Input: dimensioned drawing with shaded views. Units: mm. Origin: part minimum x, y, z. A direction names the side the tool comes from. Round coordinates to 2 decimals unless told otherwise and drop trailing zeros. Loops run counter-clockwise (first coordinate to the right, second up) from the corner with the lowest first, then second, coordinate; pieces in that order, holes last. Notation, with made-up numbers: (-5.5, 58.5) - (21.5, 58.5) arc R19 ccw to (21.5, 95.5) - close; hole circle Ø3 at (12, 8). An arc over 180 degrees is marked (long way). One line per question, with ' | ' between items. Start each with the question number.
Item 1: Material intervals for line 1 along Y through (x, z) = (24, 7.75); line 2 along Z through (x, y) = (26.5, 18), sorted ascending.
Item 2: Section C-C, the plane y = 5.75. Return loops of the section in (x, z).
Item 3: Section B-B, the plane z = 13.25. Return loops of the section in (x, y).
Item 4: First-contact query: pin 1 (10 mm diameter, centred on x = 17, y = 3, fed in from -Z); pin 2 (2 mm diameter, centred on x = 23, z = 13, fed in from -Y); pin 3 (7.5 mm diameter, centred on x = 17.5, z = 10, fed in from +Y). Flat tips, straight axial feed; report the tip coordinate or a pass-through.
Item 5: Set-up query: the marked faces 1, 2 and 3. Return all of +Z, -Z, +X, -X, +Y, -Y with unobstructed straight access to the full face (end or side cutting, diameter ignored); none if empty.
Item 6: Section A-A, the plane x = 19.5. Return loops of the section in (y, z), plus the area to 4 significant figures.
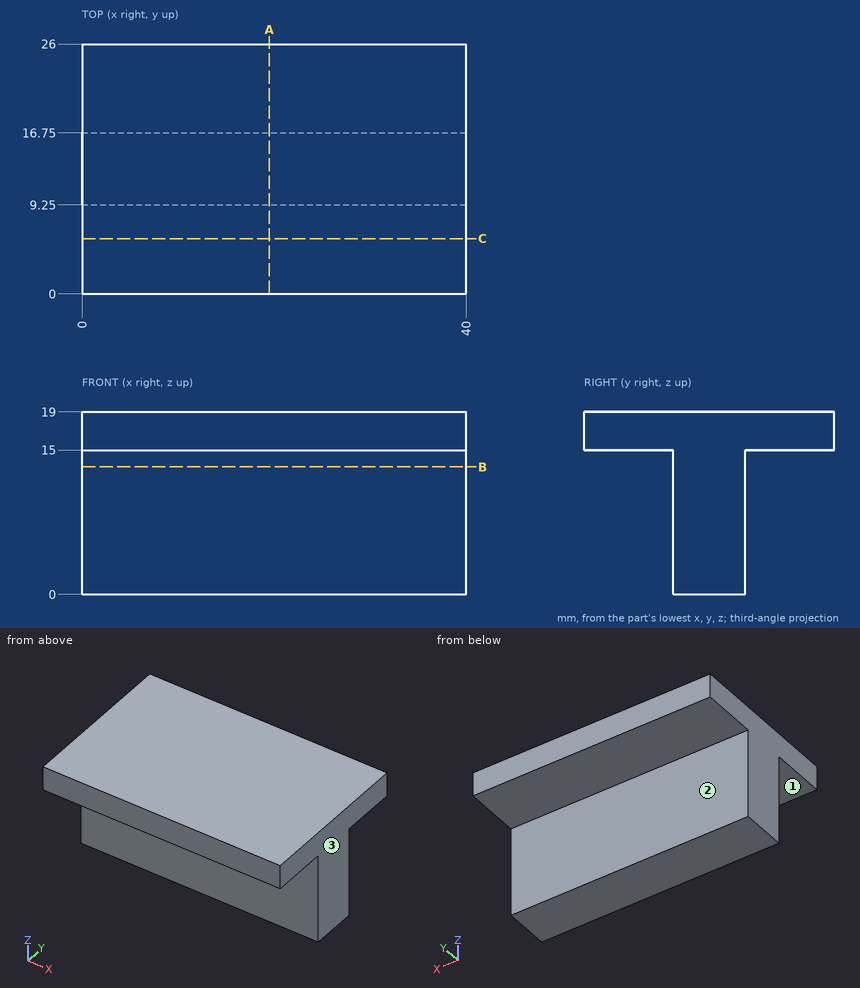
Return value:
1) line 1: 9.25 to 16.75 | line 2: 15 to 19
2) outline: (0, 15) - (40, 15) - (40, 19) - (0, 19) - close
3) outline: (0, 9.25) - (40, 9.25) - (40, 16.75) - (0, 16.75) - close
4) pin 1: z = 15 | pin 2: y = 9.25 | pin 3: y = 16.75
5) face 1: -Z, +X, -X, -Y | face 2: -Z, +X, -X, +Y | face 3: +Z, -Z, +X, +Y, -Y
6) outline: (0, 15) - (9.25, 15) - (9.25, 0) - (16.75, 0) - (16.75, 15) - (26, 15) - (26, 19) - (0, 19) - close | area: 216.5 mm2
